```python
from build123d import *

# Parameters (mm, degrees)
FILLET2_R        = 0.2
LPATTERN10_COUNT = 20
LPATTERN10_PITCH = 0.25


with BuildPart() as part:
    # Sketch1 → Revolve1 (revolve)
    with BuildSketch(Plane(origin=(0, 0, 0), x_dir=(1, 0, 0), z_dir=(0, 1, 0))):
        with BuildLine():
            Line((2.37, 1.5), (13.37, 1.5))
            Line((13.37, 1.5), (13.37, 0))
            Line((13.37, 0), (0, 0))
            ThreePointArc((0, 0), (0.224879408, 1.215980768), (0.869770135, 2.271109163))
            ThreePointArc((0.869770135, 2.271109163), (1.549177667, 2.754228297), (2.37, 2.9))
            Line((2.37, 2.9), (2.37, 1.5))
        make_face()
    revolve(axis=Axis((-13.629268293, 0, 0), (1, 0, 0)))

    # Fillet2
    fillet2_edges = [part.edges().sort_by_distance(p)[0] for p in [
        (2.37, 0, 1.5),
    ]]
    fillet(fillet2_edges, radius=FILLET2_R)

    # Sketch4 → Cut-Revolve1 (revolve, cut)
    with BuildSketch(Plane(origin=(0, 0, 0), x_dir=(1, 0, 0), z_dir=(0, 1, 0))):
        Polygon((14.103454633, 0), (14.103454633, 21), (7.743066959, 21), (13.37, 0), align=None)
    revolve(axis=Axis((4.782773752, 0, 0), (1, 0, 0)), mode=Mode.SUBTRACT)

    # Sketch2 → Cut-Loft1 section 0
    with BuildSketch(Plane(origin=(0, 0, 0), x_dir=(0, 0, -1), z_dir=(1, 0, 0)), mode=Mode.PRIVATE) as cut_loft1_s0:
        Polygon((-0.4625, 0.4625), (-1.85, 0.4625), (-1.85, -0.4625), (-0.4625, -0.4625), (-0.4625, -1.85), (0.4625, -1.85), (0.4625, -0.4625), (1.85, -0.4625), (1.85, 0.4625), (0.4625, 0.4625), (0.4625, 1.85), (-0.4625, 1.85), align=None)
    loft([Vertex(2.62, 0, 0), cut_loft1_s0.sketch], mode=Mode.SUBTRACT)

    # Sketch6 → Cut-Revolve10 (revolve, cut)
    with BuildSketch(Plane.XY):
        Polygon((8.37, 1.7), (8.495, 1.7), (8.495, 1.5), (8.4325, 1.391746825), (8.37, 1.5), align=None)
    cut_revolve10 = revolve(axis=Axis((10.774329131, 0, 0), (-1, 0, 0)), mode=Mode.SUBTRACT)

    # LPattern10: Cut-Revolve10 ×20
    with Locations(*[(i * LPATTERN10_PITCH, 0, 0) for i in range(1, LPATTERN10_COUNT)]):
        add(cut_revolve10, mode=Mode.SUBTRACT)


solid = part.part
```
Geometry: final body of the model. Coordinates: model frame, mm. A direction names the side the tool comes from. Give positions to 0.01 mm unless a question says otherwise; leave off trailing zeros. Loops run counter-clockwise (first coordinate to the right, second up) from the corner with the lowest first, then second, coordinate; pieces in that order, holes last. Notation, with made-up numbers: (-4.75, 5) -> (4.25, 5) arc R18 ccw to (4.25, 32) -> close; hole circle Ø2 at (13.25, 23). An arc over 180 degrees is marked (long way). Return JSON: item names as keys, results as strings.
Item 1: Mould query, pull axis Z, two halves, no side actions, for faces 3 (the flat face through (1.04, -0.28, 0.62)), 4 (the flat face through (1.04, 0.28, -0.62)), 5 (the cylindrical face through (5.51, 0.45, -1.43)). Classes: released by +Z, released by -Z, zero draft, split by the parting line, or undercut.
Filled in:
{"face 3": "undercut", "face 4": "undercut", "face 5": "split by the parting line"}
Item 2: Line query: line 1 (Y direction, x = 3.5, z = 0.05); line 2 (Z direction, x = 8.25, y = 0.3); line 3 (Z direction, x = 7.25, y = -0.6). Output: solid intervals per line, ascending.
Filled in:
{"line 1": "-1.5 to 1.5", "line 2": "-1.47 to 1.47", "line 3": "-1.37 to 1.37"}
Item 3: Section A-A, the plane x = 3.5. Output: boundary loops of the cut face in (y, z), plus the area to 3 significant figures.
Filled in:
{"outline": "circle Ø3 at (0, 0)", "area": "7.07 mm^2"}
Item 4: Pin query (flat end, axial travel): P1, Ø2, axis at x = 4, y = -0.5, coming from the +Z side; P2, Ø1, axis at x = 3, z = -0.5, coming from the -Y side; P3, Ø1, axis at x = 2.5, y = -2.5, coming from the -Z side; P4, Ø1.5, axis at y = 0.5, z = 0, coming from the +X side. Return the tip coordinate at first contact, or that it passes through.
Filled in:
{"P1": "z = 1.5", "P2": "y = -1.5", "P3": "z = -2.08", "P4": "x = 13.37"}
Item 5: Access query for faces 1 (the flat face through (1.24, -0.005, -0.974)), 2 (the conical face through (13.35, -0.06, -0.03)). Directions: +Z, -Z, +X, -X, +Y, -Y. A direction counts if a zero-diameter tool reaches every point of the face in a straight line with its end or side. Return the directions, or none.
Filled in:
{"face 1": "-X", "face 2": "+X"}
